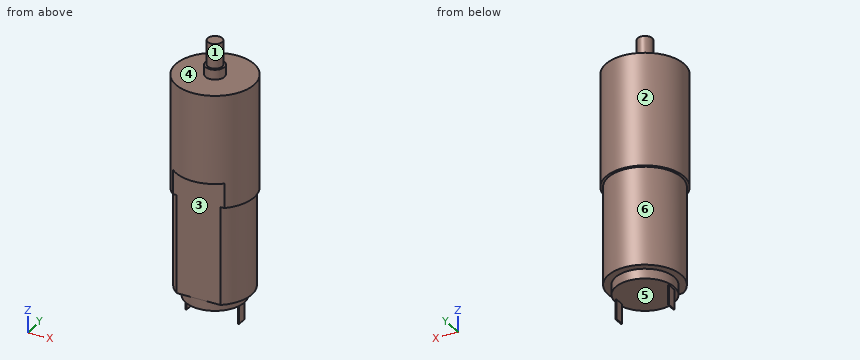
from build123d import *

# Parameters (mm, degrees)
SKETCH_1_R          = 8
EXTRUDE_1_DEPTH     = 23
SKETCH_2_R          = 6
EXTRUDE_2_DEPTH     = 22
SKETCH_4_R          = 1.95
EXTRUDE_4_DEPTH     = 2
SKETCH_5_R          = 7.5
EXTRUDE_6_DEPTH     = 20
CUT_EXTRUDE_2_DEPTH = 25
SKETCH_7_W          = 0.238746812
SKETCH_7_H          = 2.029347906
SKETCH_7_W_2        = 0.208903461
EXTRUDE_7_DEPTH     = 4
SKETCH_8_R          = 1.5
EXTRUDE_8_DEPTH     = 5


with BuildPart() as part:
    # 草图1 → 凸台-拉伸1 (new body)
    with BuildSketch(Plane.XY):
        Circle(SKETCH_1_R)
    extrude(amount=EXTRUDE_1_DEPTH)

    # 草图2 → 凸台-拉伸2 (add)
    with BuildSketch(Plane(origin=(0, 0, 0), x_dir=(-1, 0, 0), z_dir=(0, 0, -1))):
        Circle(SKETCH_2_R)
    extrude(amount=EXTRUDE_2_DEPTH)

    # 草图4 → 凸台-拉伸4 (add)
    with BuildSketch(Plane.XY.offset(23)):
        Circle(SKETCH_4_R)
    extrude(amount=EXTRUDE_4_DEPTH)

    # 草图5 → 凸台-拉伸6 (add)
    with BuildSketch(Plane(origin=(0, 0, 0), x_dir=(-1, 0, 0), z_dir=(0, 0, -1))):
        with Locations(Location((0, 0, 0), (0, 0, 180))):
            Circle(SKETCH_5_R)
    extrude(amount=EXTRUDE_6_DEPTH)

    # 草图6 → 切除-拉伸2 (cut)
    with BuildSketch(Plane(origin=(0, 0, -20), x_dir=(-1, 0, 0), z_dir=(0, 0, -1))):
        Polygon((0, -6), (7.251934426, -6), (7.251934426, -9), (-7.072874317, -9), (-7.072874317, -6), align=None)
    extrude(amount=-CUT_EXTRUDE_2_DEPTH, mode=Mode.SUBTRACT)

    # 草图7 → 凸台-拉伸7 (add)
    with BuildSketch(Plane(origin=(0, 0, -22), x_dir=(-1, 0, 0), z_dir=(0, 0, -1))):
        with Locations((-5.40164663, 0)):
            Rectangle(SKETCH_7_W, SKETCH_7_H)
        with Locations((5.371803278, 0)):
            Rectangle(SKETCH_7_W_2, SKETCH_7_H)
    extrude(amount=EXTRUDE_7_DEPTH)

    # 草图8 → 凸台-拉伸8 (add)
    with BuildSketch(Plane.XY.offset(25)):
        Circle(SKETCH_8_R)
    extrude(amount=EXTRUDE_8_DEPTH)


solid = part.part
The listing builds one solid part. Answer for the finished solid, in the listing's coordinates (mm). Face numbers are marked on the shaded views. A direction names the side the tool comes from. Round coordinates to 2 decimals unless told otherwise and drop trailing zeros. Write each loop counter-clockwise with the first axis right and the second up, starting at its lowest first coordinate (ties: lowest second). Pieces come first, ordered by that corner, then holes. Notation, with made-up numbers: (-21.75, -7) - (5.25, -7) arc R17 ccw to (5.25, 5) - close; hole circle Ø8 at (24, 65). An arc over 180 degrees is marked (long way). Use a Markdown table: item, result. Add a question column.
1. A tool of negligible diameter and unlimited length cuts with its end or side. For the marked faces 1, 2 and 3, from which of +Z, -Z, +X, -X, +Y, -Y can it reach the whole face along a straight path? Write none if from no direction.
2. The part is cut by section C-C (z = 23.5). Write down the section's boundary in (x, y), and give its area (3 significant figures).
3. The part is cut by section B-B (x = 3). Write down the section's boundary in (y, z).
4. The part is cut by section A-A (y = 0). Write down the section's boundary in (x, z), and give its area (3 significant figures).
5. The part is cut by section D-D (x = -6.5). Write down the section's boundary in (y, z), and give its area (3 significant figures).
6. Consider line 1 (Z direction, x = -2.25, y = -5.75); line 2 (Z direction, x = -1.5, y = 1); line 3 (Y direction, x = 1.5, z = -12.5). Determine where each line is inside the solid, lowest interval first.
7. Flat-ended cylindrical pins translate along their axes: P1, Ø4, axis at x = -0.5, y = 5.5, coming from the -Z side; P2, Ø1.6, axis at y = 0, z = -23, coming from the -X side; P3, Ø3, axis at x = -5, z = -13.5, coming from the +Y side. Find the tip coordinate at first contact, or state that the pin passes through.
8. For a pull along X with two mould halves and no side action, classify the marked faces 4, 5 and 6 as +X half, -X half, draft (parallel to the pull), parting line (faces both ways), or undercut.
Reported:
| question | item | result |
|---|---|---|
| 1 | face 1 | +Z |
| 1 | face 2 | +Z, -Z |
| 1 | face 3 | -Z, +X, -X, -Y |
| 2 | outline | circle Ø3.9 at (0, 0) |
| 2 | area | 11.9 mm^2 |
| 3 | outline | (-7.42, 5) - (-6, 5) - (-6, -20) - (-5.2, -20) - (-5.2, -22) - (5.2, -22) - (5.2, -20) - (6.87, -20) - (6.87, 0) - (7.42, 0) - (7.42, 23) - (-7.42, 23) - close |
| 4 | outline | (-8, 0) - (-7.5, 0) - (-7.5, -20) - (-6, -20) - (-6, -22) - (-5.48, -22) - (-5.48, -26) - (-5.27, -26) - (-5.27, -22) - (5.28, -22) - (5.28, -26) - (5.52, -26) - (5.52, -22) - (6, -22) - (6, -20) - (7.5, -20) - (7.5, 0) - (8, 0) - (8, 23) - (1.95, 23) - (1.95, 25) - (1.5, 25) - (1.5, 30) - (-1.5, 30) - (-1.5, 25) - (-1.95, 25) - (-1.95, 23) - (-8, 23) - close |
| 4 | area | 717 mm^2 |
| 5 | outline | (-4.66, 0) - (-3.74, 0) - (-3.74, -20) - (3.74, -20) - (3.74, 0) - (4.66, 0) - (4.66, 23) - (-4.66, 23) - close |
| 5 | area | 364 mm^2 |
| 6 | line 1 | -20 to 23 |
| 6 | line 2 | -22 to 25 |
| 6 | line 3 | -6 to 7.35 |
| 7 | P1 | z = -22 |
| 7 | P2 | x = -5.48 |
| 7 | P3 | y = 6.63 |
| 8 | face 4 | draft |
| 8 | face 5 | undercut |
| 8 | face 6 | parting line |
